Work out the finished part from the listing and answer in its coordinate system (mm). A direction names the side the tool comes from. Coordinates: 2 decimals unless noted, no trailing zeros. Loops run counter-clockwise (first coordinate to the right, second up) from the corner with the lowest first, then second, coordinate; pieces in that order, holes last. Notation, with made-up numbers: (47.25, 4.5) -> (68.25, 4.5) arc R14 cw to (68.25, 18.5) -> close; hole circle Ø1 at (-16, -32.75). An arc over 180 degrees is marked (long way). Use a Markdown table: item, result.
from build123d import *

# Parameters (mm, degrees)
SKETCH_W        = 82
SKETCH_H        = 40
PAD_DEPTH       = 1.2
SKETCH001_W     = 5.5
SKETCH001_H     = 8
PAD001_DEPTH    = 15
SKETCH002_R     = 1.5
POCKET_DEPTH    = 40.001
SKETCH003_W     = 1.6
SKETCH003_H     = 35
PAD002_DEPTH    = 10
SKETCH004_R     = 3
SKETCH004_R_2   = 1.5
PAD003_DEPTH    = 4
SKETCH005_R     = 1.7
POCKET001_DEPTH = 1.201
SKETCH006_R     = 1.5
POCKET002_DEPTH = 1.201
SKETCH007_W     = 1.6
SKETCH007_H     = 8
POCKET003_DEPTH = 10


with BuildPart() as part:
    # Sketch → Pad (new body)
    with BuildSketch(Plane.XY):
        with Locations((41, 20)):
            Rectangle(SKETCH_W, SKETCH_H)
    extrude(amount=PAD_DEPTH)

    # Sketch001 (on Face6 of Pad) → Pad001 (join)
    with BuildSketch(Plane.XY.offset(1.2)):
        with Locations((2.75, 4)):
            Rectangle(SKETCH001_W, SKETCH001_H)
        with Locations((79.25, 4)):
            Rectangle(SKETCH001_W, SKETCH001_H)
    extrude(amount=PAD001_DEPTH)

    # Sketch002 (on Face5 of Pad001) → Pocket (cut, through all)
    with BuildSketch(Plane.XZ):
        with Locations((2.75, 13.7)):
            Circle(SKETCH002_R)
        with Locations((2.75, 4.5)):
            Circle(SKETCH002_R)
        with Locations((79.25, 13.7)):
            Circle(SKETCH002_R)
        with Locations((79.25, 4.5)):
            Circle(SKETCH002_R)
    extrude(amount=-POCKET_DEPTH, mode=Mode.SUBTRACT)

    # Sketch003 (on Face6 of Pocket) → Pad002 (join)
    with BuildSketch(Plane.XY.offset(1.2)):
        with Locations((26.2, 22.5)):
            Rectangle(SKETCH003_W, SKETCH003_H)
        with Locations((54.2, 22.5)):
            Rectangle(SKETCH003_W, SKETCH003_H)
    extrude(amount=PAD002_DEPTH)

    # Sketch004 (on Face6 of Pad002) → Pad003 (join)
    with BuildSketch(Plane.XY.offset(1.2)):
        with Locations((10.7, 26.5)):
            Circle(SKETCH004_R)
        with Locations((10.7, 26.5)):
            Circle(SKETCH004_R_2, mode=Mode.SUBTRACT)
    extrude(amount=PAD003_DEPTH)

    # Sketch005 (on Face6 of Pad003) → Pocket001 (cut, through all)
    with BuildSketch(Plane.XY.offset(1.2)):
        with Locations((5, 35)):
            Circle(SKETCH005_R)
        with Locations((77, 35)):
            Circle(SKETCH005_R)
        with Locations((69, 5)):
            Circle(SKETCH005_R)
        with Locations((13, 5)):
            Circle(SKETCH005_R)
    extrude(amount=-POCKET001_DEPTH, mode=Mode.SUBTRACT)

    # Sketch006 (on Face38 of Pocket001) → Pocket002 (cut, through all)
    with BuildSketch(Plane.XY.offset(1.2)):
        with Locations((10.7, 26.5)):
            Circle(SKETCH006_R)
    extrude(amount=-POCKET002_DEPTH, mode=Mode.SUBTRACT)

    # Sketch007 (on Face36 of Pocket002) → Pocket003 (cut)
    with BuildSketch(Plane.XY.offset(11.2)):
        with Locations((26.2, 36)):
            Rectangle(SKETCH007_W, SKETCH007_H)
    extrude(amount=-POCKET003_DEPTH, mode=Mode.SUBTRACT)


solid = part.part
Q1. Section D-D on y = 18.5 is taken. Determine the outline of the cut face in (x, z), and give its area (3 significant figures).
Solved:
| item | result |
|---|---|
| outline | (0, 0) -> (82, 0) -> (82, 1.2) -> (55, 1.2) -> (55, 11.2) -> (53.4, 11.2) -> (53.4, 1.2) -> (27, 1.2) -> (27, 11.2) -> (25.4, 11.2) -> (25.4, 1.2) -> (0, 1.2) -> close |
| area | 130 mm² |
Q2. For faces 1 (the flat face through (25.4, 18, 6)), 2 (the flat face through (54, 5, 6)), 3 (the cylindrical face through (13.47, 25.35, 3.17)), determine the directions among +Z, -Z, +X, -X, +Y, -Y from which every point of the face is accessible in a straight line to the end or side of a thin tool.
Solved:
| item | result |
|---|---|
| face 1 | +Z, +Y, -Y |
| face 2 | +Z, -Y |
| face 3 | +Z |
Q3. Section B-B on z = 13.7 is taken. Determine the outline of the cut face in (x, y).
Solved:
| item | result |
|---|---|
| outline | (0, 0) -> (1.25, 0) -> (1.25, 8) -> (0, 8) -> close; (4.25, 0) -> (5.5, 0) -> (5.5, 8) -> (4.25, 8) -> close; (76.5, 0) -> (77.75, 0) -> (77.75, 8) -> (76.5, 8) -> close; (80.75, 0) -> (82, 0) -> (82, 8) -> (80.75, 8) -> close |
Q4. Section A-A on x = 69 is taken. Determine the outline of the cut face in (y, z), and give its area (3 significant figures).
Solved:
| item | result |
|---|---|
| outline | (0, 0) -> (3.3, 0) -> (3.3, 1.2) -> (0, 1.2) -> close; (6.7, 0) -> (40, 0) -> (40, 1.2) -> (6.7, 1.2) -> close |
| area | 43.9 mm² |
Q5. Section C-C on y = 35 is taken. Determine the outline of the cut face in (x, z).
Solved:
| item | result |
|---|---|
| outline | (0, 0) -> (3.3, 0) -> (3.3, 1.2) -> (0, 1.2) -> close; (6.7, 0) -> (75.3, 0) -> (75.3, 1.2) -> (55, 1.2) -> (55, 11.2) -> (53.4, 11.2) -> (53.4, 1.2) -> (6.7, 1.2) -> close; (78.7, 0) -> (82, 0) -> (82, 1.2) -> (78.7, 1.2) -> close |
Q6. Determine the mould class of faces 4 (the flat face through (5.5, 4, 9)), 5 (the flat face through (79, 4, 16.2)), 6 (the cylindrical face through (80.68, 3.94, 14.15)) for opening direction Z: pulls with the +Z half, pulls with the -Z half, needs draft (parallel to the pull), parting line crosses it, or undercut.
Solved:
| item | result |
|---|---|
| face 4 | needs draft |
| face 5 | pulls with the +Z half |
| face 6 | undercut |
Q7. Given pin 1 Ø1.3 at (x, y) = (54.5, 24) entering from +Z; pin 2 Ø6 at (x, z) = (3.5, 10) entering from +Y; pin 3 Ø1.8 at (x, z) = (54, 4) entering from -Y, each flat-ended and moving along its own axis, determine where each tip first touches the part or whether it passes through.
Solved:
| item | result |
|---|---|
| pin 1 | z = 11.2 |
| pin 2 | y = 8 |
| pin 3 | y = 5 |
Q8. Consider line 1 (Z direction, x = 2.75, y = 6); line 2 (X direction, y = 23, z = 9.75); line 3 (Y direction, x = 5, z = 0.25). Determine where each line is inside the solid, lowest interval first. Write a range as [from, to].
Solved:
| item | result |
|---|---|
| line 1 | [0, 3], [6, 12.2], [15.2, 16.2] |
| line 2 | [25.4, 27], [53.4, 55] |
| line 3 | [0, 33.3], [36.7, 40] |
